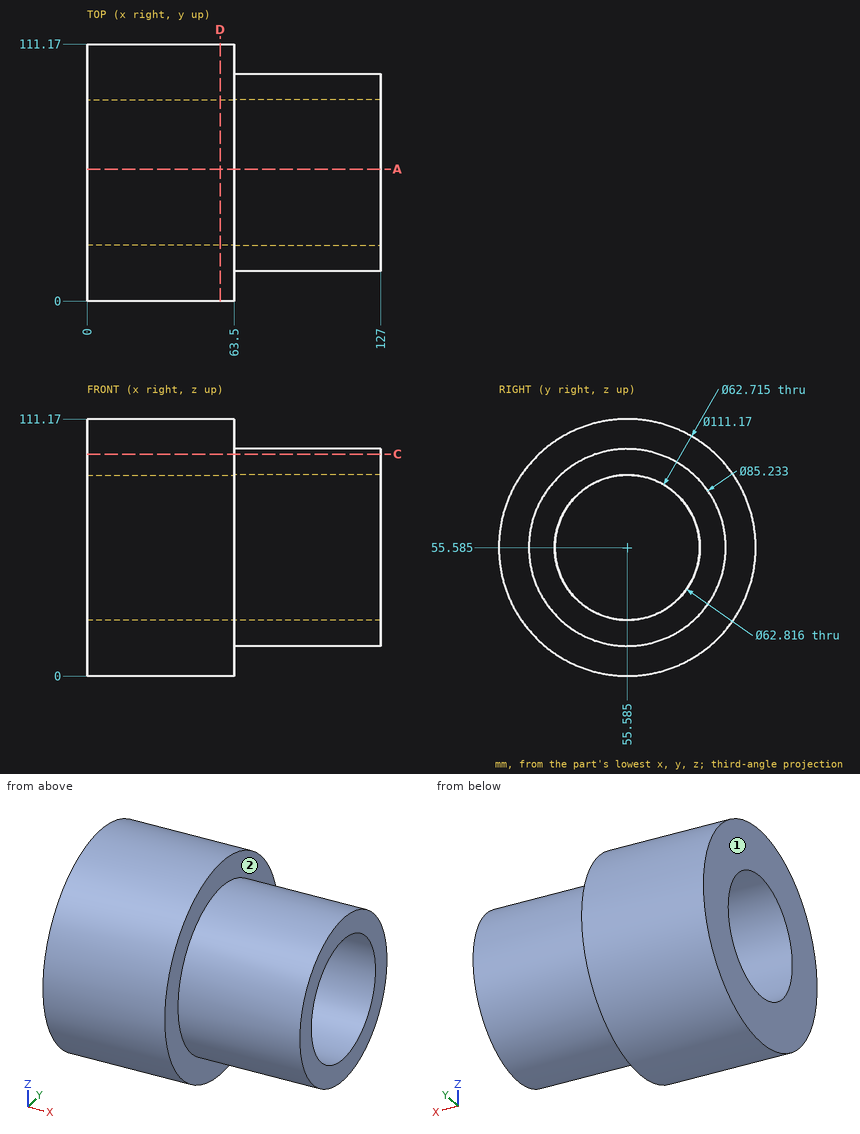
Part print with two shaded views. Sizes in mm from the minimum x, y, z corner. A direction names the side the tool comes from. Coordinates: 2 decimals unless noted, no trailing zeros. Write each loop counter-clockwise with the first axis right and the second up, starting at its lowest first coordinate (ties: lowest second). Pieces come first, ordered by that corner, then holes. Notation, with made-up numbers: (86, 84) - (129, 84) arc R32 ccw to (129, 114) - close; hole circle Ø1 at (-5.5, 62). An arc over 180 degrees is marked (long way). One line per item, written item: value. Start each with the question number.
1. Tool access for the marked faces 1 and 2: list every direction of +Z, -Z, +X, -X, +Y, -Y with a clear straight run to the whole face (end or side of a thin tool).
2. Probe line 1 (Z direction, x = 121, y = 54.5) (1 decimal); line 2 (Z direction, x = 15.5, y = 72); line 3 (Y direction, x = 82, z = 82) (1 decimal). List the from-to ranges inside material, lowest first. Write a range as from..to.
3. Slice it at A-A (y = 57). Write the cut outline in (x, z).
4. Slice it at D-D (x = 57.5). Write the cut outline in (y, z) (1 decimal).
5. Slice it at C-C (z = 96). Write the cut outline in (x, y) (1 decimal), plus the area to 3 significant figures.
6. Flat gauge pins, fed straight in: pin 1 (3 mm diameter, centred on x = 106, z = 84, fed in from +Y); pin 2 (1 mm diameter, centred on x = 56, z = 41.5, fed in from -Y); pin 3 (10 mm diameter, centred on x = 49.5, z = 70, fed in from +Y). Where does each tip first touch, or does it go through?
Answers below:
1. face 1: +Z, -Z, -X, +Y, -Y
1. face 2: +X
2. line 1: z = 13..24.2, 87..98.2
2. line 2: z = 2.48..28.87, 82.3..108.69
2. line 3: y = 22.1..38.6, 72.6..89
3. outline: (0, 0.02) - (63.5, 0.02) - (63.5, 12.99) - (127, 12.99) - (127, 24.21) - (63.5, 24.21) - (63.5, 24.26) - (0, 24.26) - close; (0, 86.91) - (63.5, 86.91) - (63.5, 86.96) - (127, 86.96) - (127, 98.18) - (63.5, 98.18) - (63.5, 111.15) - (0, 111.15) - close
4. outline: circle Ø111.2 at (55.6, 55.6); hole circle Ø62.7 at (55.6, 55.6)
5. outline: (0, 17.4) - (63.5, 17.4) - (63.5, 42.1) - (127, 42.1) - (127, 69.1) - (63.5, 69.1) - (63.5, 93.7) - (0, 93.7) - close
5. area: 6,560 mm^2
6. pin 1: stops at y = 88.63
6. pin 2: stops at y = 1.69
6. pin 3: stops at y = 110.37
